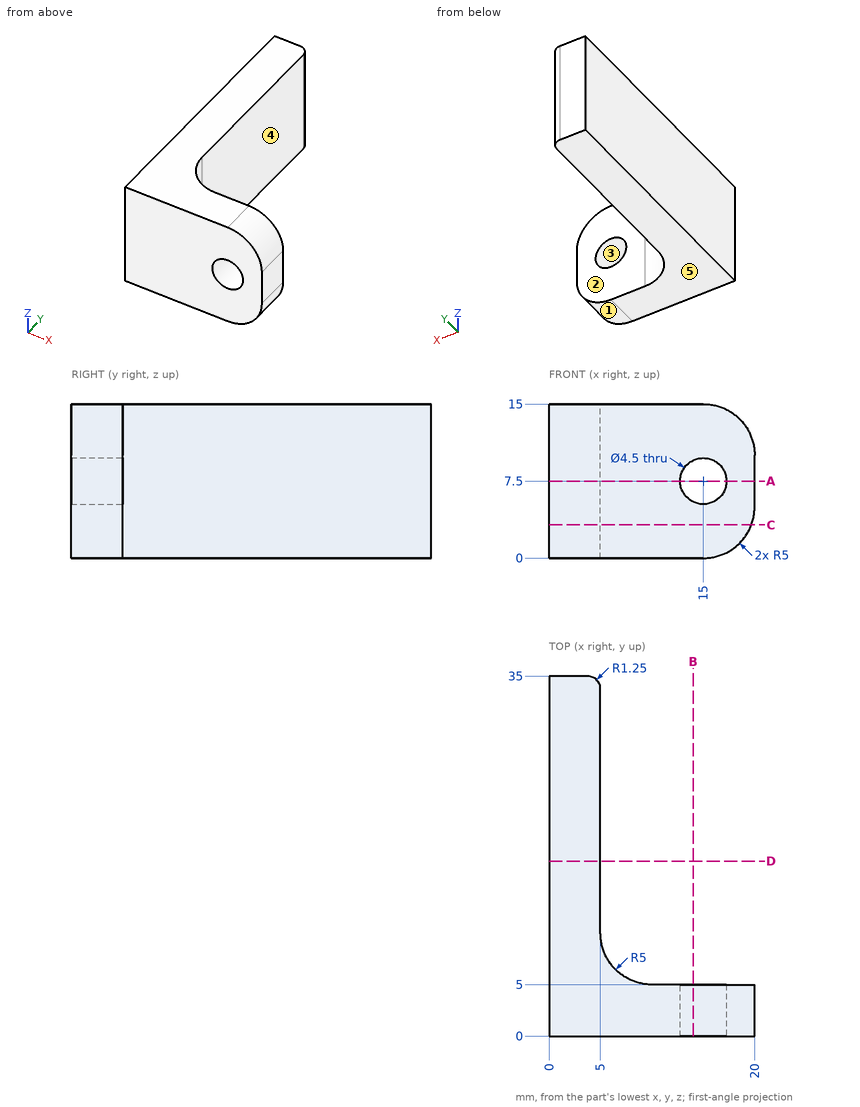
Geometry: see drawing. Coordinates: mm, zero at the bounding-box minimum. A direction names the side the tool comes from. Coordinates: 2 decimals unless noted, no trailing zeros. Write each loop counter-clockwise with the first axis right and the second up, starting at its lowest first coordinate (ties: lowest second). Pieces come first, ordered by that corner, then holes.
1) Section D-D on y = 17. Output: boundary loops of the cut face in (x, z), and give its area (3 significant figures).
2) Set-up query: the marked faces 1 and 2. Return all of +Z, -Z, +X, -X, +Y, -Y with unobstructed straight access to the full face (end or side cutting, diameter ignored); none if empty.
3) Material intervals for line 1 along Z through (x, y) = (15, 3.8); line 2 along X through (y, z) = (23, 1.5), sorted ascending.
4) Section C-C on z = 3.25. Output: boundary loops of the cut face in (x, y), and give its area (3 significant figures).
5) Mould query, pull axis X, two halves, no side actions, for the marked faces 3, 4 and 5. Classes: pulls with the +X half, pulls with the -X half, needs draft (parallel to the pull), parting line crosses it, or undercut.
6) Section A-A on z = 7.5. Output: boundary loops of the cut face in (x, y).
7) Section B-B on x = 14. Output: boundary loops of the cut face in (y, z).
8) Pin query (flat end, axial travel): pin 1 Ø7 at (x, z) = (15, 7.5) entering from +Y; pin 2 Ø7.5 at (y, z) = (22, 9) entering from +X. Return the tip coordinate at first contact, or that it passes through.
Check result:
1. outline: (0, 0) - (5, 0) - (5, 15) - (0, 15) - close
1. area: 75.0 mm2
2. face 1: -Z, +X, +Y, -Y
2. face 2: +Z, -Z, +X, +Y
3. line 1: z = 0 to 5.25, 9.75 to 15
3. line 2: x = 0 to 5
4. outline: (0, 0) - (19.68, 0) - (19.68, 5) - (10, 5) arc R5 cw to (5, 10) - (5, 33.75) arc R1.25 ccw to (3.75, 35) - (0, 35) - close
4. area: 253 mm2
5. face 3: undercut
5. face 4: pulls with the +X half
5. face 5: needs draft
6. outline: (0, 0) - (12.75, 0) - (12.75, 5) - (10, 5) arc R5 cw to (5, 10) - (5, 33.75) arc R1.25 ccw to (3.75, 35) - (0, 35) - close; (17.25, 0) - (20, 0) - (20, 5) - (17.25, 5) - close
7. outline: (0, 0) - (5, 0) - (5, 5.48) - (0, 5.48) - close; (0, 9.52) - (5, 9.52) - (5, 15) - (0, 15) - close
8. pin 1: stops at y = 5
8. pin 2: stops at x = 5
